from build123d import *

# Parameters (mm, degrees)
BOSS_EXTRUDE1_DEPTH      = 21.59
BOSS_EXTRUDE1_DEPTH_BACK = 21.59
BOSS_EXTRUDE2_DEPTH      = 6.35
BOSS_EXTRUDE2_DEPTH_BACK = 6.35
SKETCH1_4_W              = 6.35
SKETCH1_4_H              = 3.81
SKETCH3_W                = 26.67
SKETCH3_H                = 31.242
BOSS_EXTRUDE3_DEPTH      = 3.81
SKETCH4_R                = 1.524
CUT_EXTRUDE1_DEPTH       = 2.286
SKETCH4_4_R              = 1.524
CUT_EXTRUDE3_DEPTH       = 39.616354359
SKETCH6_W                = 7.62
SKETCH6_H                = 7.62
CUT_EXTRUDE4_DEPTH       = 48.910486994
FILLET1_R                = 2.54
FILLET2_R                = 1.27
CHAMFER1_SIZE            = 1.27
CHAMFER2_SIZE            = 0.254


with BuildPart() as part:
    # Sketch1 → Boss-Extrude1 (new, two sides: drawn at the far end of the back side and taken through both)
    with BuildSketch(Plane(origin=(0, 0, 0), x_dir=(1, 0, 0), z_dir=(0, 1, 0)).offset(-BOSS_EXTRUDE1_DEPTH_BACK)):
        Polygon((-16.51, 31.242), (-16.51, 0), (10.16, 0), (10.16, 3.81), (-12.7, 3.81), (-12.7, 27.432), (10.16, 27.432), (10.16, 31.242), align=None)
    extrude(amount=BOSS_EXTRUDE1_DEPTH + BOSS_EXTRUDE1_DEPTH_BACK)

    # Sketch1<4> → Boss-Extrude2 (add, two sides: drawn at the far end of the back side and taken through both)
    with BuildSketch(Plane(origin=(0, 0, 0), x_dir=(1, 0, 0), z_dir=(0, 1, 0)).offset(-BOSS_EXTRUDE2_DEPTH_BACK)):
        with Locations((13.335, 1.905)):
            Rectangle(SKETCH1_4_W, SKETCH1_4_H)
    extrude(amount=BOSS_EXTRUDE2_DEPTH + BOSS_EXTRUDE2_DEPTH_BACK)

    # Sketch3 → Boss-Extrude3 (add)
    with BuildSketch(Plane(origin=(0, 21.59, 0), x_dir=(1, 0, 0), z_dir=(0, 1, 0))):
        with Locations((-3.175, 15.621)):
            Rectangle(SKETCH3_W, SKETCH3_H)
    boss_extrude3 = extrude(amount=-BOSS_EXTRUDE3_DEPTH)

    # Mirror1: Boss-Extrude3 across plane
    add(boss_extrude3.mirror(Plane.ZX))

    # Sketch4 → Cut-Extrude1 (cut)
    with BuildSketch(Plane.XY.offset(-27.432)):
        Polygon((0.3556, 15.426316158), (-1.0033, 17.78), (-3.7211, 17.78), (-5.08, 15.426316158), (-3.7211, 13.072632315), (-1.0033, 13.072632315), align=None)
        with Locations((-2.3622, 15.426316158)):
            Circle(SKETCH4_R, mode=Mode.SUBTRACT)
    cut_extrude1 = extrude(amount=-CUT_EXTRUDE1_DEPTH, mode=Mode.SUBTRACT)

    # Sketch4<4> → Cut-Extrude3 (cut, through all)
    with BuildSketch(Plane.XY.offset(-27.432)):
        with Locations((-2.3622, 15.426316158)):
            Circle(SKETCH4_4_R)
    cut_extrude3 = extrude(amount=-CUT_EXTRUDE3_DEPTH, mode=Mode.SUBTRACT)

    # Mirror2: Cut-Extrude1, Cut-Extrude3 across plane
    add(cut_extrude1.mirror(Plane.ZX), mode=Mode.SUBTRACT)
    add(cut_extrude3.mirror(Plane.ZX), mode=Mode.SUBTRACT)

    # Sketch6 → Cut-Extrude4 (cut, through all)
    with BuildSketch(Plane(origin=(-12.7, 0, 0), x_dir=(0, 0, -1), z_dir=(1, 0, 0))):
        with Locations((23.622, -13.97)):
            Rectangle(SKETCH6_W, SKETCH6_H)
    extrude(amount=-CUT_EXTRUDE4_DEPTH, mode=Mode.SUBTRACT)

    # Fillet1
    fillet1_edges = [part.edges().sort_by_distance(p)[0] for p in [
        (-16.51, 0, 0),
        (-16.51, 21.59, -15.621),
        (-3.175, 21.59, 0),
        (-16.51, -21.59, -15.621),
        (-3.175, -21.59, 0),
    ]]
    fillet(fillet1_edges, radius=FILLET1_R)

    # Fillet2
    fillet2_edges = [part.edges().sort_by_distance(p)[0] for p in [
        (-16.51, -13.97, -27.432),
        (-16.51, -17.78, -23.622),
        (-16.51, -13.97, -19.812),
        (-16.51, -10.16, -23.622),
        (-12.7, -10.16, -23.622),
        (-12.7, -13.97, -19.812),
    ]]
    fillet(fillet2_edges, radius=FILLET2_R - 0.0001)  # a hair under: the kernel refuses the full size

    # Chamfer1
    chamfer1_edges = [part.edges().sort_by_distance(p)[0] for p in [
        (13.335, -6.35, -3.81),
        (16.51, 0, -3.81),
        (16.51, -6.35, -1.905),
        (13.335, 6.35, -3.81),
        (16.51, 6.35, -1.905),
    ]]
    chamfer(chamfer1_edges, length=CHAMFER1_SIZE)

    # Chamfer2
    chamfer2_edges = [part.edges().sort_by_distance(p)[0] for p in [
        (-3.8862, 15.426316158, -31.242),
        (-3.8862, -15.426316158, -31.242),
    ]]
    chamfer(chamfer2_edges, length=CHAMFER2_SIZE)


solid = part.part
The model under review builds one solid part; all positions refer to its coordinate system, in mm. A direction names the side the tool comes from. Coordinates: 2 decimals unless noted, no trailing zeros. Loops run counter-clockwise (first coordinate to the right, second up) from the corner with the lowest first, then second, coordinate; pieces in that order, holes last. Notation, with made-up numbers: (24, -11) -> (28, -11) arc R29 ccw to (28, 20) -> close; hole circle Ø11 at (-8.75, 85). An arc over 180 degrees is marked (long way). Use a Markdown table: item, result. Add a question column.
1. Add section C-C on y = -11.5. Write out the cut boundary in (x, z), plus the area to 3 significant figures.
2. Draft analysis for pull direction X (two halves, no side actions). For faces 1 (the face through (16.51, 0, -1)), 2 (the face through (-2.561, -16.937, -30.344)), 3 (the face through (-15.786, -20.826, -16.69)), state which applies: pulls with the +X half, pulls with the -X half, needs draft (parallel to the pull), parting line crosses it, or undercut.
3. To check wall thickness, follow line 1 (Z direction, x = -4.5, y = -14); line 2 (Y direction, x = -10, z = -16); line 3 (X direction, y = 16, z = -12). State the ranges of each line that lie inside material, in increasing order.
4. Add section B-B on x = 5. Write out the cut boundary in (y, z), plus the area to 3 significant figures.
5. Add section D-D on z = -17.5. Write out the cut boundary in (x, y), plus the area to 3 significant figures.
6. Machinability: for faces 4 (the face through (-2, 0, -27.432)), 5 (the face through (13, 6.35, -1)), 6 (the face through (-16.148, -13.899, -27.814)), 7 (the face through (-1, -17, -29.718)), which of the approach directions +Z, -Z, +X, -X, +Y, -Y give a long, thin tool a straight path to every point of the face, cutting with its end or side? Answer none if there is none.
7. Clearance check with flat-ended pins moving along their axes: pin 1 Ø8 at (y, z) = (-12, -19.5) entering from +X; pin 2 Ø3 at (x, z) = (12, -1.5) entering from -Y; pin 3 Ø1.3 at (x, z) = (12, -1.5) entering from +Y. State where each tip first meets the part, or that it passes through.
Returned:
| question | item | result |
|---|---|---|
| 1 | outline | (-16.51, -31.24) -> (10.16, -31.24) -> (10.16, -27.43) -> (-15.24, -27.43) arc R1.27 ccw to (-16.51, -28.7) -> close; (-16.51, -18.54) arc R1.27 ccw to (-15.24, -19.81) -> (-13.97, -19.81) arc R1.27 ccw to (-12.7, -18.54) -> (-12.7, -3.81) -> (10.16, -3.81) -> (10.16, 0) -> (-13.97, 0) arc R2.54 ccw to (-16.51, -2.54) -> close |
| 1 | area | 262 mm² |
| 2 | face 1 | pulls with the +X half |
| 2 | face 2 | undercut |
| 2 | face 3 | pulls with the -X half |
| 3 | line 1 | z = -31.24 to -27.43, -3.81 to 0 |
| 3 | line 2 | y = -21.59 to -17.78, 17.78 to 21.59 |
| 3 | line 3 | x = -16.51 to -12.7 |
| 4 | outline | (-21.59, -31.24) -> (21.59, -31.24) -> (21.59, -2.54) arc R2.54 ccw to (19.05, 0) -> (-19.05, 0) arc R2.54 ccw to (-21.59, -2.54) -> close; hole (-17.78, -27.43) -> (17.78, -27.43) -> (17.78, -3.81) -> (-17.78, -3.81) -> close |
| 4 | area | 506 mm² |
| 5 | outline | (-16.51, -19.05) arc R2.54 ccw to (-13.97, -21.59) -> (10.16, -21.59) -> (10.16, -17.78) -> (-12.7, -17.78) -> (-12.7, 17.78) -> (10.16, 17.78) -> (10.16, 21.59) -> (-13.97, 21.59) arc R2.54 ccw to (-16.51, 19.05) -> close |
| 5 | area | 336 mm² |
| 6 | face 4 | +X |
| 6 | face 5 | +Z, -Z, +X, +Y |
| 6 | face 6 | -X |
| 6 | face 7 | none |
| 7 | pin 1 | stops at x = -12.7 |
| 7 | pin 2 | stops at y = -6.35 |
| 7 | pin 3 | stops at y = 6.35 |
